The model under review builds one solid part; all positions refer to its coordinate system, in mm. Face numbers are marked on the shaded views. A direction names the side the tool comes from. Give positions to 0.01 mm unless a question says otherwise; leave off trailing zeros. Order: outer loops, then holes, each group sorted by start corner. A loop starts at its lowest first (then second) coordinate and runs counter-clockwise, first axis right, second up. Notation, with made-up numbers: (-13, 55.25) -> (29, 55.25) arc R33 cw to (29, 86.25) -> close; hole circle Ø9 at (43, 69). An arc over 180 degrees is marked (long way). Use one line per item in the form item = value.
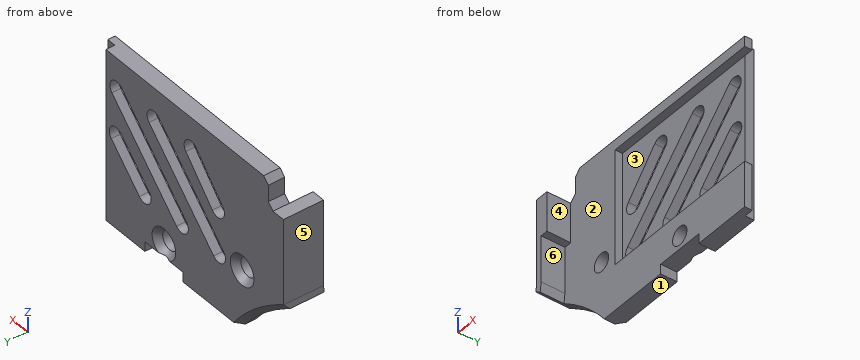
```python
from build123d import *

# Parameters (mm, degrees)
SKETCH_221_R           = 1.55
EXTRUDE_926_DEPTH      = 2.75
SKETCH_1005_W          = 35.000000002
SKETCH_1005_H          = 4.75
EXTRUDE_1111_DEPTH     = 2.75
EXTRUDE_1_DEPTH        = 2.75
F_2_PCB_START          = -4
F_2_PCB_DEPTH          = 4
SKETCH_2154_W          = 1.5
SKETCH_2154_H          = 28.99988509
EXTRUDE_2226_DEPTH     = 1.25
SKETCH_2278_W          = 27.915979255
SKETCH_2278_H          = 19.5
PCB_DEPTH              = 1.25
CUT_EXTRUDE_2_DEPTH    = 33.528299963
CHAMFER_1_SIZE         = 1
CHAMFER_2_SIZE         = 1
CUT_EXTRUDE_3384_DEPTH = 4


with BuildPart() as part:
    # Sketch 221 → Extrude 926 (new body)
    with BuildSketch(Plane(origin=(0, 0, 0), x_dir=(1, 0, 0), z_dir=(0, 1, 0))):
        with BuildLine():
            ThreePointArc((-16.252981126, 10), (-20.15501929, 5.688743466), (-24.715186194, 2.08073674))
            Line((-24.715186194, 2.08073674), (-24.500000002, 0.312480077))
            Line((-24.500000002, 0.312480077), (-24.500000002, -7.263629174))
            Line((-24.500000002, -7.263629174), (-22.500000002, -7.263629174))
            Line((-22.500000002, -7.263629174), (-22.500000002, -14.24988509))
            Line((-22.500000002, -14.24988509), (12.5, -14.24988509))
            Line((12.5, -14.24988509), (12.5, 10))
            Line((12.5, 10), (4.100927374, 10))
            Line((4.100927374, 10), (4.100927374, 8.35804307))
            Line((4.100927374, 8.35804307), (-4.100927378, 8.35804307))
            Line((-4.100927378, 8.35804307), (-4.100927378, 10))
            Line((-4.100927378, 10), (-16.252981126, 10))
        make_face()
        with Locations(Location((-16.865979255, 0, 0), (0, 0, 270))):
            Circle(SKETCH_221_R, mode=Mode.SUBTRACT)
        with Locations(Location((-2e-09, 6.108043073, 0), (0, 0, 270))):
            Circle(SKETCH_221_R, mode=Mode.SUBTRACT)
    extrude(amount=EXTRUDE_926_DEPTH)

    # Sketch 1005 → Extrude 1111 (add)
    with BuildSketch(Plane(origin=(0, 0, 0), x_dir=(1, 0, 0), z_dir=(0, 1, 0))):
        with Locations((-5.000000001, -16.62488509)):
            Rectangle(SKETCH_1005_W, SKETCH_1005_H)
    extrude(amount=EXTRUDE_1111_DEPTH)

    # Sketch 1191 → 卡榫结构-1 (add)
    with BuildSketch(Plane(origin=(0, 0, 0), x_dir=(1, 0, 0), z_dir=(0, 1, 0))):
        with BuildLine():
            Line((-25.750000002, -14.213629174), (-22.500000002, -14.213629174))
            Line((-22.500000002, -14.213629174), (-22.500000002, -7.263629174))
            Line((-22.500000002, -7.263629174), (-24.500000002, -7.263629174))
            Line((-24.500000002, -7.263629174), (-24.500000002, 0.312480077))
            Line((-24.500000002, 0.312480077), (-24.715186194, 2.08073674))
            ThreePointArc((-24.715186194, 2.08073674), (-25.291636518, 1.705823535), (-25.875319612, 1.342273079))
            Line((-25.875319612, 1.342273079), (-25.750000002, 0.312480077))
            Line((-25.750000002, 0.312480077), (-25.750000002, -14.213629174))
        make_face()
    extrude(amount=EXTRUDE_1_DEPTH)

    # 草图5<4> → 卡榫结构-2-注意PCB凸出部分 (add)
    with BuildSketch(Plane(origin=(0, 0, 0), x_dir=(1, 0, 0), z_dir=(0, 1, 0)).offset(F_2_PCB_START)):
        with BuildLine():
            Line((-25.750000002, -14.213629174), (-23.500000002, -14.213629174))
            Line((-23.500000002, -14.213629174), (-23.500000002, -7.263629174))
            Line((-23.500000002, -7.263629174), (-24.500000002, -7.263629174))
            Line((-24.500000002, -7.263629174), (-24.500000002, 0.312480077))
            Line((-24.500000002, 0.312480077), (-24.715186194, 2.08073674))
            ThreePointArc((-24.715186194, 2.08073674), (-25.291636518, 1.705823535), (-25.875319612, 1.342273079))
            Line((-25.875319612, 1.342273079), (-25.750000002, 0.312480077))
            Line((-25.750000002, 0.312480077), (-25.750000002, -14.213629174))
        make_face()
    extrude(amount=F_2_PCB_DEPTH)

    # Sketch 2154 → Extrude 2226 (add)
    with BuildSketch(Plane(origin=(0, 0, 0), x_dir=(1, 0, 0), z_dir=(0, 1, 0))):
        with Locations((13.25, -4.499942545)):
            Rectangle(SKETCH_2154_W, SKETCH_2154_H)
    extrude(amount=EXTRUDE_2226_DEPTH)

    # Sketch 2278 → 稳压PCB器件高度补偿 (cut)
    with BuildSketch(Plane(origin=(0, 0, 0), x_dir=(1, 0, 0), z_dir=(0, 1, 0))):
        with Locations((0.042010372, -7.5)):
            Rectangle(SKETCH_2278_W, SKETCH_2278_H)
    extrude(amount=PCB_DEPTH, mode=Mode.SUBTRACT)

    # Sketch 2514 → 切除-拉伸2 (cut, through all)
    with BuildSketch(Plane.XZ.offset(-1.25)):
        with BuildLine():
            Line((3.173198201, 0.69066828), (9.20694903, 6.724419109))
            ThreePointArc((9.20694903, 6.724419109), (11.328269373, 6.724419109), (11.328269373, 4.603098766))
            Line((11.328269373, 4.603098766), (5.294518544, -1.430652063))
            ThreePointArc((5.294518544, -1.430652063), (3.173198201, -1.430652063), (3.173198201, 0.69066828))
        make_face()
        with BuildLine():
            Line((-4.826801799, 0.69066828), (9.08250112, 14.5999712))
            ThreePointArc((9.08250112, 14.5999712), (11.203821464, 14.5999712), (11.203821464, 12.478650856))
            Line((11.203821464, 12.478650856), (-2.705481456, -1.430652063))
            ThreePointArc((-2.705481456, -1.430652063), (-4.826801799, -1.430652063), (-4.826801799, 0.69066828))
        make_face()
        with BuildLine():
            Line((-12.826801799, 0.69066828), (1.08250112, 14.5999712))
            ThreePointArc((1.08250112, 14.5999712), (3.203821464, 14.5999712), (3.203821464, 12.478650856))
            Line((3.203821464, 12.478650856), (-10.705481456, -1.430652063))
            ThreePointArc((-10.705481456, -1.430652063), (-12.826801799, -1.430652063), (-12.826801799, 0.69066828))
        make_face()
        with BuildLine():
            Line((-4.738916917, 12.539185601), (-10.437516852, 6.169395501))
            ThreePointArc((-10.437516852, 6.169395501), (-12.555564069, 6.051599138), (-12.673360433, 8.169646355))
            Line((-12.673360433, 8.169646355), (-6.974760498, 14.539436455))
            ThreePointArc((-6.974760498, 14.539436455), (-4.856713281, 14.657232819), (-4.738916917, 12.539185601))
        make_face()
    extrude(amount=-CUT_EXTRUDE_2_DEPTH, mode=Mode.SUBTRACT)

    # 倒角1
    chamfer_1_edges = [part.edges().sort_by_distance(p)[0] for p in [
        (-20.661675073, 2.75, -5.223818951),
        (-22.500000002, 1.375, 18.99988509),
        (-22.500000002, 1.375, 14.213629174),
    ]]
    chamfer(chamfer_1_edges, length=CHAMFER_1_SIZE)

    # 倒角2
    # the kernel refuses this chamfer: 1 mm, written as the material it takes off along each edge
    with BuildSketch(Plane(origin=(-2e-09, 2.75, -6.108043073), x_dir=(0, 0, 1), z_dir=(-1, 0, 0))) as chamfer_2_piece_1:
        Polygon((1.55 + CHAMFER_2_SIZE, 0), (1.55, -CHAMFER_2_SIZE), (1.55, 0), align=None)
    revolve(axis=Axis((-2e-09, 2.75, -6.108043073), (0, 1, 0)), mode=Mode.SUBTRACT)
    with BuildSketch(Plane(origin=(-16.865979255, 2.75, 0), x_dir=(0, 0, 1), z_dir=(-1, 0, 0))) as chamfer_2_piece_2:
        Polygon((1.55 + CHAMFER_2_SIZE, 0), (1.55, -CHAMFER_2_SIZE), (1.55, 0), align=None)
    revolve(axis=Axis((-16.865979255, 2.75, 0), (0, 1, 0)), mode=Mode.SUBTRACT)

    # 草图1 → Cut-Extrude 3384 (cut)
    with BuildSketch(Plane.XZ.offset(4)):
        with BuildLine():
            Line((-24.715186194, -2.08073674), (-24.500000002, -0.312480077))
            Line((-24.500000002, -0.312480077), (-24.500000002, 7.263629174))
            Line((-24.500000002, 7.263629174), (-23.500000002, 7.263629174))
            Line((-23.500000002, 7.263629174), (-23.500000002, 7.513629174))
            Line((-23.500000002, 7.513629174), (-24.750000002, 7.513629174))
            Line((-24.750000002, 7.513629174), (-24.750000002, -0.312480077))
            Line((-24.750000002, -0.312480077), (-24.946632534, -1.928275128))
            ThreePointArc((-24.946632534, -1.928275128), (-24.830758909, -2.004277534), (-24.715186194, -2.08073674))
        make_face()
    extrude(amount=-CUT_EXTRUDE_3384_DEPTH, mode=Mode.SUBTRACT)


solid = part.part
```
1. Add section A-A on y = -3.5. Give the boundary of the cut face in (x, z), then the cut area to 3 significant figures.
Values:
outline = (-25.88, -1.34) arc R35.11 cw to (-24.95, -1.93) -> (-24.75, -0.31) -> (-24.75, 7.51) -> (-23.5, 7.51) -> (-23.5, 14.21) -> (-25.75, 14.21) -> (-25.75, -0.31) -> close
area = 24.2 mm^2
2. Tool access review of the marked faces 4, 5 and 6: name each direction out of +Z, -Z, +X, -X, +Y, -Y from which nothing blocks a thin tool from reaching the whole face with its end or side.
Values:
face_4 = +Z, -Z, +X, -Y
face_5 = +Z, -X, +Y, -Y
face_6 = -Z, +X, -Y
3. For pin 1 Ø2 at (y, z) = (1, 17) entering from -X; pin 2 Ø3 at (x, y) = (-0.5, 1.5) entering from -Z; pin 3 Ø2 at (y, z) = (1, 0) entering from -X; pin 4 Ø12 at (x, z) = (0, 4) entering from +Y, all flat-tipped, find the tip position at first contact; note any pin that passes through.
Values:
pin_1 = -22.5
pin_2 = -8.36
pin_3 = -25.83
pin_4 = 2.75
4. For L1, parallel to Z at x = 0, y = 0.7; L2, parallel to X at y = 0.8, z = 0; L3, parallel to X at y = 1.75, z = -1, list the stretches that pass through material, from the lowest coordinate up.
Values:
L1 = -8.36 to -7.66, -4.56 to -2.25, 17.25 to 19
L2 = -25.75 to -18.42, -15.32 to -13.92
L3 = -25.83 to -18.05, -15.68 to -13.13, -10.27 to -5.13, -2.27 to 2.87, 5.73 to 12.5
5. Add section B-B on z = 13.75. Give the boundary of the cut face in (x, y).
Values:
outline = (-25.75, -4) -> (-23.5, -4) -> (-23.5, 0) -> (-13.92, 0) -> (-13.92, 1.25) -> (-7.68, 1.25) -> (-7.68, 2.75) -> (-25.75, 2.75) -> close; (-4.37, 1.25) -> (0.23, 1.25) -> (0.23, 2.75) -> (-4.37, 2.75) -> close; (3.63, 1.25) -> (8.23, 1.25) -> (8.23, 2.75) -> (3.63, 2.75) -> close; (11.63, 1.25) -> (12.5, 1.25) -> (12.5, 2.75) -> (11.63, 2.75) -> close
6. Add section D-D on x = -6.5. Give the boundary of the cut face in (y, z).
Values:
outline = (0, -10) -> (2.75, -10) -> (2.75, 2.77) -> (1.25, 2.77) -> (1.25, -2.25) -> (0, -2.25) -> close; (0, 17.25) -> (1.25, 17.25) -> (1.25, 14.89) -> (2.75, 14.89) -> (2.75, 19) -> (0, 19) -> close; (1.25, 7.02) -> (2.75, 7.02) -> (2.75, 10.57) -> (1.25, 10.57) -> close
7. The part is to be moulded in two halves that separate along Z. For the marked faces 1, 2 and 3, say which applies: +Z half, -Z half, draft (parallel to the pull), parting line (faces both ways), or undercut.
Values:
face_1 = -Z half
face_2 = draft
face_3 = undercut
8. Add section C-C on x = 0. Give the boundary of the cut face in (y, z).
Values:
outline = (0, -8.36) -> (2.45, -8.36) -> (1.75, -7.66) -> (0, -7.66) -> close; (0, -4.56) -> (1.75, -4.56) -> (2.75, -3.56) -> (2.75, 1.27) -> (1.25, 1.27) -> (1.25, -2.25) -> (0, -2.25) -> close; (0, 17.25) -> (1.25, 17.25) -> (1.25, 13.52) -> (2.75, 13.52) -> (2.75, 19) -> (0, 19) -> close; (1.25, 5.52) -> (2.75, 5.52) -> (2.75, 9.27) -> (1.25, 9.27) -> close
